from build123d import *

# Parameters (mm, degrees)
EXTRUDE_1_DEPTH = 3
SKETCH_2_R      = 2.25
EXTRUDE_2_DEPTH = 1
SKETCH_3_R      = 3
EXTRUDE_3_DEPTH = 1
FILLET_1_R      = 1


with BuildPart() as part:
    # 草图1 → 凸台-拉伸1 (new body)
    with BuildSketch(Plane.XY):
        Polygon((0, 0), (4.5, 0), (2.25, 3.897114317), align=None)
    extrude(amount=EXTRUDE_1_DEPTH)

    # 草图2 → 凸台-拉伸2 (add)
    with BuildSketch(Plane.XY.offset(3)):
        with Locations(Location((2.25, 1.299038106, 0), (0, 0, 204.735610317))):
            Circle(SKETCH_2_R)
    extrude(amount=EXTRUDE_2_DEPTH)

    # 草图3 → 凸台-拉伸3 (add)
    with BuildSketch(Plane.XY.offset(4)):
        with Locations((2.25, 1.299038106)):
            Circle(SKETCH_3_R)
    extrude(amount=EXTRUDE_3_DEPTH)

    # 圆角1
    # the kernel refuses this fillet: 1 mm, written as the material it takes off along each edge
    with BuildSketch(Plane(origin=(2.25, 3.897114317, -4.330127019), x_dir=(-0.4999999999999997, -0.8660254037844388, 0), z_dir=(0, 0, 1))) as fillet_1_piece_1:
        with BuildLine():
            CenterArc((FILLET_1_R * 1.73205080757, FILLET_1_R), FILLET_1_R, 150, 120)
            Line((FILLET_1_R * 0.866025403784, FILLET_1_R * 1.5), (0, 0))
            Line((0, 0), (FILLET_1_R * 1.73205080757, 0))
        make_face()
    extrude(amount=7.330127019, mode=Mode.SUBTRACT)
    with BuildSketch(Plane(origin=(4.5, 0, -4.330127019), x_dir=(-1, 0, 0), z_dir=(0, 0, 1)), Plane(origin=(0, 0, -4.330127019), x_dir=(0.49999999999999983, 0.8660254037844387, 0), z_dir=(0, 0, 1))) as fillet_1_piece_2:
        with BuildLine():
            CenterArc((FILLET_1_R * 1.73205080757, -FILLET_1_R), FILLET_1_R, 90, 120)
            Line((FILLET_1_R * 0.866025403784, -FILLET_1_R * 1.5), (0, 0))
            Line((0, 0), (FILLET_1_R * 1.73205080757, 0))
        make_face()
    extrude(amount=7.330127019, mode=Mode.SUBTRACT)


solid = part.part
Can you work these out from the model? Positions are in its coordinate system, mm. A direction names the side the tool comes from. Coordinates: 2 decimals unless noted, no trailing zeros. Loops run counter-clockwise (first coordinate to the right, second up) from the corner with the lowest first, then second, coordinate; pieces in that order, holes last. Notation, with made-up numbers: M -23,59.5 L -18,59.5 A26 cw -18,80.5 Z; hole C 22.5,20 d11. An arc over 180 degrees is marked long. Answer as CSV lines item,"result". Start each with the question number.
1. Suppose I cut it at D-D, the plane x = 4.4. List the corners of the cut face in (y, z) for me.
2. Suppose I cut it at A-A, the plane z = 1.9. List the corners of the cut face in (x, y) for me, plus the area to 3 significant figures.
3. Suppose I cut it at C-C, the plane y = 0.45. List the corners of the cut face in (x, z) for me, plus the area to 3 significant figures.
4. If I drill on probe 1 along Z at (x, y) = (3.8, 2.3); probe 2 along Z at (x, y) = (-0.1, 0.6); probe 3 along Y at (x, z) = (2.3, 3.4), over which ranges is the centre line in solid material (lowest first)? Write a range as [from, to].
5. For pin 1 Ø1.5 at (x, z) = (1.5, 1.5) entering from +Y; pin 2 Ø1.5 at (y, z) = (2, 1) entering from -X, each with a flat end and sliding along its axis, tell me the tip position at first contact or that it passes through.
6. For faces 1 (the face through (2, 0, 1)), 2 (the face through (0.86, 0.51, 1.48)), 3 (the face through (2.265, 2.897, 1.479)), 4 (the face through (4, 2, 3)), which set-ups out of +Z, -Z, +X, -X, +Y, -Y let a thin tool reach every point of the face, with its end or its side?
7. Suppose I cut it at B-B, the plane x = 2.25. List the corners of the cut face in (y, z) for me, plus the area to 3 significant figures.
Output:
1,outline,"M -0.79,4 L 0.64,4 L 0.64,3 L 1.96,3 L 1.96,4 L 3.39,4 L 3.39,5 L -0.79,5 Z"
2,outline,"M 0.87,1.5 A1 ccw 1.73,0 L 2.77,0 A1 ccw 3.63,1.5 L 3.12,2.4 A1 ccw 1.38,2.4 Z"
2,area,"6.71 mm^2"
3,outline,"M -0.63,4 L 0.17,4 L 0.17,3 L 0.9,3 L 0.9,0 L 3.6,0 L 3.6,3 L 4.33,3 L 4.33,4 L 5.13,4 L 5.13,5 L -0.63,5 Z"
3,area,"18.0 mm^2"
4,probe 1,"z = [3, 5]"
4,probe 2,"z = [4, 5]"
4,probe 3,"y = [-0.95, 3.55]"
5,pin 1,"stops at y = 2.9"
5,pin 2,"stops at x = 0.76"
6,face 1,"-Z, +X, -X, -Y"
6,face 2,"-Z, -X"
6,face 3,"-Z, +Y"
6,face 4,"-Z"
7,outline,"M -1.7,4 L -0.95,4 L -0.95,3 L 0,3 L 0,0 L 2.9,0 L 2.9,3 L 3.55,3 L 3.55,4 L 4.3,4 L 4.3,5 L -1.7,5 Z"
7,area,"19.2 mm^2"
